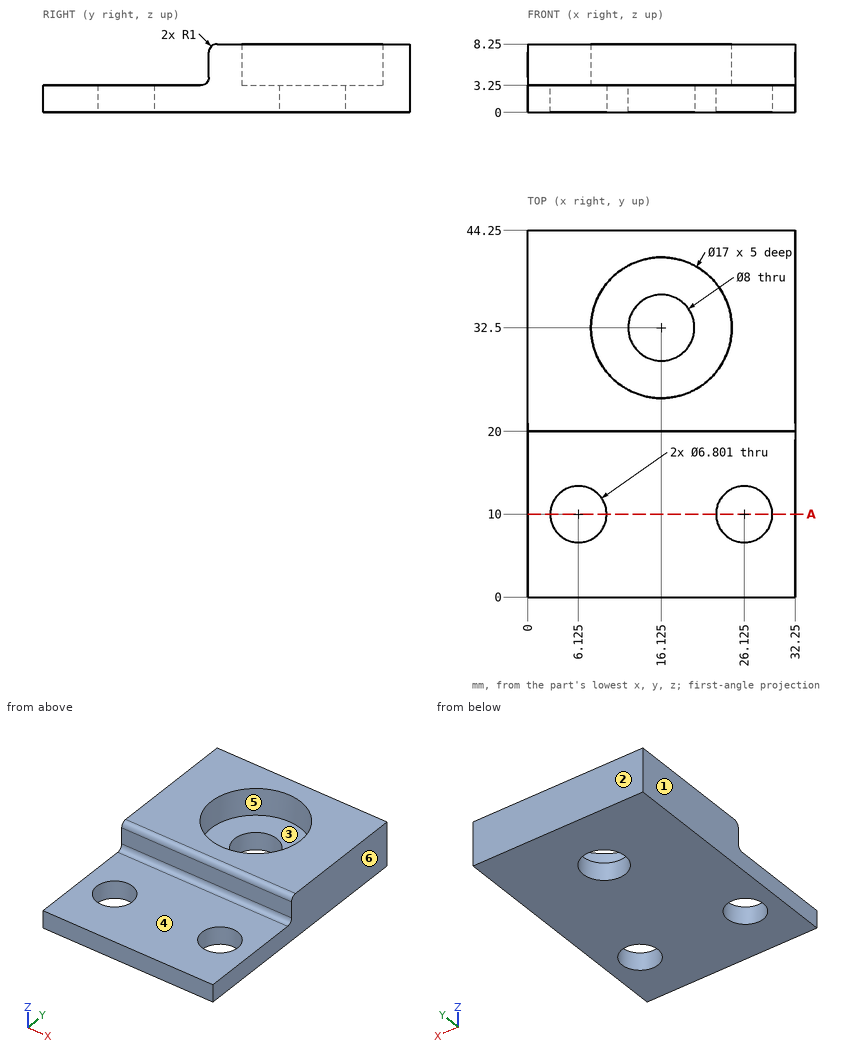
Print and shaded views of the part. All mm, measured from the part's lowest x, y and z. A direction names the side the tool comes from. Round coordinates to 2 decimals unless told otherwise and drop trailing zeros.
Q1. Which spindle directions (+Z, -Z, +X, -X, +Y, -Y) get a long thin tool onto all of the face, cutting with end or side? Do the marked faces 4, 5 and 6. Say none if no direction does.
Q2. Two-plate mould, pull along Y, no slides. Class the marked faces 1, 2 and 3: pulls with the +Y half, pulls with the -Y half, needs draft (parallel to the pull), parting line crosses it, or undercut.
Q3. Wall check: L1, parallel to Y at x = 26.5, z = 2; L2, parallel to Y at x = 7, z = 6.5; L3, parallel to Y at x = 11, z = 7. Give the ranges that are in metal, low to high.
Q4. Drop flat-ended pins along their axis: pin 1 (8 mm diameter, centred on x = 19.5, y = 25, fed in from -Z); pin 2 (8.5 mm diameter, centred on x = 18, y = 33.5, fed in from +Z); pin 3 (2.5 mm diameter, centred on x = 20.5, z = 5, fed in from -Y); pin 4 (3 mm diameter, centred on x = 3.5, z = 5.5, fed in from -Y). Give the stop position or say it passes through.
Q5. Slice it at A-A (y = 10). State how many separate pieces and enclosed holes the cut face has, and give its area (3 significant figures).
Results below:
1. face 4: +Z, +X, -X, -Y
1. face 5: +Z
1. face 6: +Z, -Z, +X, +Y, -Y
2. face 1: needs draft
2. face 2: pulls with the +Y half
2. face 3: undercut
3. L1: y = 0 to 6.62, 13.38 to 44.25
3. L2: y = 20 to 44.25
3. L3: y = 20 to 25.72, 39.28 to 44.25
4. pin 1: stops at z = 0
4. pin 2: stops at z = 3.25
4. pin 3: stops at y = 19.87
4. pin 4: stops at y = 19.97
5. separate pieces: 3
5. enclosed holes: 0
5. area: 60.6 mm2
